```python
from build123d import *

# Parameters (mm, degrees)
SKETCH2_W                      = 12
SKETCH2_H                      = 18
EXTRUDE1_DEPTH                 = 31.75
EXTRUDE1_2_DEPTH               = 31.75
SKETCH4_R                      = 9.5885
MAGNET_CAVITY_DEPTH            = 44.163207712
SKETCH18_W                     = 1.25
SKETCH18_H                     = 30
M3X0_5_TAPPED_HOLE1_AT_2_COUNT = 2
M3X0_5_TAPPED_HOLE1_AT_2_PITCH = 9
M3X0_5_TAPPED_HOLE1_AT_3_COUNT = 2
M3X0_5_TAPPED_HOLE1_AT_3_PITCH = 25.395037131
M3_CLEARANCE_HOLE1_AT_2_COUNT  = 2
M3_CLEARANCE_HOLE1_AT_2_PITCH  = 21.091007592
EXTRUDE3_DEPTH                 = 44.163207712
EXTRUDE5_DEPTH                 = 4.5
EXTRUDE8_START                 = -8
EXTRUDE8_DEPTH                 = 36.406015976
CIRPATTERN1_COUNT              = 3


with BuildPart() as part:
    # Sketch2 → Extrude1 (new body)
    with BuildSketch(Plane(origin=(0, 4.5, 0), x_dir=(-1, 0, 0), z_dir=(0, 1, 0))):
        with Locations((9, 1.982307478)):
            Rectangle(SKETCH2_W, SKETCH2_H)
    extrude(amount=EXTRUDE1_DEPTH)


with BuildPart() as body_2:
    # Sketch2 → Extrude1 2 (new body)
    with BuildSketch(Plane(origin=(0, 4.5, 0), x_dir=(-1, 0, 0), z_dir=(0, 1, 0))):
        with Locations((-9, 1.982307478)):
            Rectangle(SKETCH2_W, SKETCH2_H)
    extrude(amount=EXTRUDE1_2_DEPTH)


with BuildPart() as magnet_cavity_tool:
    # Sketch4 → Magnet Cavity (new, through all)
    with BuildSketch(Plane.XY.offset(10.982307478)):
        with Locations((0.033766691, 20.375)):
            Circle(SKETCH4_R)
    extrude(amount=-MAGNET_CAVITY_DEPTH)


with BuildPart() as part_1:
    add(part.part)

    # Magnet Cavity: cut by magnet_cavity_tool
    add(magnet_cavity_tool.part, mode=Mode.SUBTRACT)


with BuildPart() as body_2_1:
    add(body_2.part)

    # Magnet Cavity: cut by magnet_cavity_tool
    add(magnet_cavity_tool.part, mode=Mode.SUBTRACT)


with BuildPart() as m3x0_5_tapped_hole1_tool:
    # Sketch18 → M3x0.5 Tapped Hole1 (revolve)
    with BuildSketch(Plane(origin=(15, 32.871578641, 6.482307478), x_dir=(0, 0, -1), z_dir=(0, 1, 0))):
        with Locations((0.625, 15)):
            Rectangle(SKETCH18_W, SKETCH18_H)
    m3x0_5_tapped_hole1 = revolve(axis=Axis((21.35, 32.871578641, 6.482307478), (-1, 0, 0)))


with BuildPart() as part_2:
    add(part_1.part)

    # M3x0.5 Tapped Hole1: cut by m3x0_5_tapped_hole1_tool
    add(m3x0_5_tapped_hole1_tool.part, mode=Mode.SUBTRACT)


with BuildPart() as body_2_2:
    add(body_2_1.part)

    # M3x0.5 Tapped Hole1: cut by m3x0_5_tapped_hole1_tool
    add(m3x0_5_tapped_hole1_tool.part, mode=Mode.SUBTRACT)


with BuildPart() as m3x0_5_tapped_hole1_at_2_tool:
    # M3x0.5 Tapped Hole1 at 2: M3x0.5 Tapped Hole1 ×2
    with Locations(*[(0, 0, -i * M3X0_5_TAPPED_HOLE1_AT_2_PITCH) for i in range(1, M3X0_5_TAPPED_HOLE1_AT_2_COUNT)]):
        add(m3x0_5_tapped_hole1)


with BuildPart() as part_3:
    add(part_2.part)

    # M3x0.5 Tapped Hole1 at 2: cut by m3x0_5_tapped_hole1_at_2_tool
    add(m3x0_5_tapped_hole1_at_2_tool.part, mode=Mode.SUBTRACT)


with BuildPart() as body_2_3:
    add(body_2_2.part)

    # M3x0.5 Tapped Hole1 at 2: cut by m3x0_5_tapped_hole1_at_2_tool
    add(m3x0_5_tapped_hole1_at_2_tool.part, mode=Mode.SUBTRACT)


with BuildPart() as m3x0_5_tapped_hole1_at_3_tool:
    # M3x0.5 Tapped Hole1 at 3: M3x0.5 Tapped Hole1 ×2
    with Locations(*[Vector(0, -0.984174866621225, -0.1771999771757721) * (i * M3X0_5_TAPPED_HOLE1_AT_3_PITCH) for i in range(1, M3X0_5_TAPPED_HOLE1_AT_3_COUNT)]):
        add(m3x0_5_tapped_hole1)


with BuildPart() as part_4:
    add(part_3.part)

    # M3x0.5 Tapped Hole1 at 3: cut by m3x0_5_tapped_hole1_at_3_tool
    add(m3x0_5_tapped_hole1_at_3_tool.part, mode=Mode.SUBTRACT)

    # Sketch24 → M3 Clearance Hole1 (revolve, cut)
    with BuildSketch(Plane(origin=(-10.511737105, 27.54122981, 10.982307478), x_dir=(0, -1, 0), z_dir=(1, 0, 0))):
        Polygon((0, 0), (0, 19.021463052), (1.7, 18), (1.7, 0), align=None)
    m3_clearance_hole1 = revolve(axis=Axis((-10.511737105, 27.54122981, 17.332307478), (0, 0, -1)), mode=Mode.SUBTRACT)



with BuildPart() as body_2_4:
    add(body_2_3.part)

    # M3x0.5 Tapped Hole1 at 3: cut by m3x0_5_tapped_hole1_at_3_tool
    add(m3x0_5_tapped_hole1_at_3_tool.part, mode=Mode.SUBTRACT)

    # M3 Clearance Hole1 at 2: M3 Clearance Hole1 ×2
    with Locations(*[(i * M3_CLEARANCE_HOLE1_AT_2_PITCH, 0, 0) for i in range(1, M3_CLEARANCE_HOLE1_AT_2_COUNT)]):
        add(m3_clearance_hole1, mode=Mode.SUBTRACT)

    # Trim Sketch → Extrude3 (cut, through all)
    with BuildSketch(Plane.XY.offset(10.982307478)):
        with BuildLine():
            Line((11, 12.456391912), (11, 4.5))
            Line((11, 4.5), (15, 4.5))
            Line((15, 4.5), (15, 36.25))
            Line((15, 36.25), (3, 36.25))
            Line((3, 36.25), (3, 35.497310661))
            Line((3, 35.497310661), (12.724200068, 35.497310661))
            Line((12.724200068, 35.497310661), (12.724200068, 30.679595884))
            ThreePointArc((12.724200068, 30.679595884), (12.757175017, 30.10630526), (12.855664924, 29.540576328))
            Line((12.855664924, 29.540576328), (14.062015368, 24.384247359))
            ThreePointArc((14.062015368, 24.384247359), (14.195982577, 20.505390111), (12.843027952, 16.867671794))
            Line((12.843027952, 16.867671794), (11.740958564, 15.075660139))
            ThreePointArc((11.740958564, 15.075660139), (11.188804349, 13.817419615), (11, 12.456391912))
        make_face()
    extrude(amount=-EXTRUDE3_DEPTH, mode=Mode.SUBTRACT)


with BuildPart() as part_5:
    add(part_4.part)

    add(body_2_4.part)  # Extrude5 merges body 2
    # Sketch1 → Extrude5 (add)
    with BuildSketch(Plane(origin=(0, 0, 0), x_dir=(1, 0, 0), z_dir=(0, 1, 0))):
        with BuildLine():
            Line((-9.989936491, 3.267692522), (-8.459547932, 0.616981784))
            Line((-8.459547932, 0.616981784), (-3.695452068, -7.634674306))
            Line((-3.695452068, -7.634674306), (-2.152576018, -10.307014014))
            ThreePointArc((-2.152576018, -10.307014014), (0.012487492, -11.557014014), (2.177551001, -10.307014014))
            Line((2.177551001, -10.307014014), (8.47827917, 0.606167299))
            Line((8.47827917, 0.606167299), (10.014911474, 3.267692522))
            ThreePointArc((10.014911474, 3.267692522), (10.014911474, 5.767692522), (7.849847964, 7.017692522))
            Line((7.849847964, 7.017692522), (4.764095865, 7.017692522))
            Line((4.764095865, 7.017692522), (-4.764095865, 7.017692522))
            Line((-4.764095865, 7.017692522), (-7.824872981, 7.017692522))
            ThreePointArc((-7.824872981, 7.017692522), (-9.989936491, 5.767692522), (-9.989936491, 3.267692522))
        make_face()
    extrude(amount=EXTRUDE5_DEPTH)

    # Sketch29 → Extrude8 (cut, through all)
    with BuildSketch(Plane(origin=(0, 0, -7.017692522), x_dir=(-1, 0, 0), z_dir=(0, 0, -1)).offset(EXTRUDE8_START)):
        Polygon((67.30851185, -64.30851185), (3, 0), (0, 3), (-3, 0), (-67.30851185, -64.30851185), (-67.30851185, -246.200451118), (67.30851185, -246.200451118), align=None)
    extrude8 = extrude(amount=-EXTRUDE8_DEPTH, mode=Mode.SUBTRACT)

    # CirPattern1: Extrude8 ×3 about axis
    cirpattern1_axis = Axis((0, 0, 1.982307478), (0, 1, 0))
    for i in range(1, CIRPATTERN1_COUNT):
        add(extrude8.rotate(cirpattern1_axis, i * 360 / CIRPATTERN1_COUNT), mode=Mode.SUBTRACT)


solid = part_5.part
```
Check sheet for the modelled part. Datum: model origin and axes. Units: mm. A direction names the side the tool comes from. Round coordinates to 2 decimals unless told otherwise and drop trailing zeros. Loops run counter-clockwise (first coordinate to the right, second up) from the corner with the lowest first, then second, coordinate; pieces in that order, holes last. Notation, with made-up numbers: M 79.25,65 L 85.25,65 A31 cw 85.25,101 Z; hole C 14,18 d5. An arc over 180 degrees is marked long. Answer as a JSON object with one key per item and string values.
1. Section check B-B (y = 16). Record the boundary of the cut face in (x, z), plus the area to 3 significant figures.
Reply:
{"outline": "M -15,-7.02 L -8.5,-7.02 L -8.5,10.98 L -15,10.98 Z; M 8.57,-7.02 L 12.31,-7.02 L 12.31,10.98 L 8.57,10.98 Z", "area": "184 mm²"}
2. Access from +Z, -Z, +X, -X, +Y, -Y to the whole of each face (thin tool, end or side, straight path). Record for faces 5 (the flat face through (-10, 20, 10.982)), 6 (the flat face through (4.618, 1.521, -2.392)), 7 (the flat face through (12.724, 33, 2)), 8 (the cylindrical face through (9.62, 20.21, 2.11)).
Reply:
{"face 5": "+Z, +X, -X, +Y, -Y", "face 6": "-Y", "face 7": "+Z, -Z, +X, +Y", "face 8": "+Z, -Z"}
3. Section check C-C (z = -4.75). State how many separate pieces and enclosed holes the cut face has, plus the area to 3 significant figures.
Reply:
{"separate pieces": "1", "enclosed holes": "2", "area": "565 mm²"}
4. Section check A-A (x = -11). Record the boundary of the cut face in (y, z).
Reply:
{"outline": "M 4.5,-7.02 L 25.91,-7.02 L 25.91,10.98 L 4.5,10.98 Z; M 29.17,-7.02 L 36.25,-7.02 L 36.25,10.98 L 29.17,10.98 Z; hole C 7.88,1.98 d2.5; hole C 32.87,-2.52 d2.5; hole C 32.87,6.48 d2.5"}
5. Mould release check, pull along Z, two halves, no side actions. Record for faces 1 (the cylindrical face through (7.794, 31.632, 6.645)), 2 (the flat face through (0.86, 2.57, 2.49)), 3 (the cylindrical face through (-11.02, 25.92, 2.11)), 4 (the cylindrical face through (9.7, 2.7, -6.2)): pulls with the +Z half, pulls with the -Z half, needs draft (parallel to the pull), parting line crosses it, or undercut.
Reply:
{"face 1": "undercut", "face 2": "undercut", "face 3": "needs draft", "face 4": "parting line crosses it"}
6. Scan lines: line 1 (X direction, y = 31, z = -1.75); line 2 (X direction, y = 9, z = -1.5); line 3 (Y direction, x = -4.75, z = 7.5). Record each from-to range of solid material in increasing order.
Reply:
{"line 1": "x = -15 to -3, 3 to 12.72", "line 2": "x = -15 to -3, 3 to 11", "line 3": "y = 4.5 to 12.07, 28.68 to 32.15, 33.6 to 36.25"}
7. Section check D-D (x = 5). Record the boundary of the cut face in (y, z).
Reply:
{"outline": "M 0,-7.02 L 12.17,-7.02 L 12.17,10.98 L 4.5,10.98 L 4.5,5.42 L 0,5.42 L 0,2.56 L 3,-0.9 L 0,-4.37 Z; M 28.58,-7.02 L 35.5,-7.02 L 35.5,10.98 L 28.58,10.98 Z; hole C 7.88,1.98 d2.5; hole C 32.87,-2.52 d2.5; hole C 32.87,6.48 d2.5"}
8. Gauge pin test, flat ends, axial feed: P1, Ø4, axis at y = 7.88, z = 1.98, coming from the +X side; P2, Ø9, axis at y = 10, z = -1, coming from the +X side; P3, Ø3.5, axis at x = -7.5, y = 16.5, coming from the +Z side; P4, Ø8, axis at x = 0, y = 18, coming from the -Z side. Record the tip position at first contact, or that the pin passes through.
Reply:
{"P1": "stops at x = 11", "P2": "stops at x = 11.44", "P3": "stops at z = 10.98", "P4": "passes through"}
